from build123d import *

# Parameters (mm, degrees)
SKETCH1_R                = 4.8387
BOSS_EXTRUDE1_DEPTH      = 25.9588
BOSS_EXTRUDE1_DEPTH_BACK = 25.9588
SKETCH2_R                = 4.8387
BOSS_EXTRUDE2_DEPTH      = 6.04901
BOSS_EXTRUDE2_DEPTH_BACK = 6.04901
SKETCH3_R                = 3.2258
CUT_EXTRUDE1_DEPTH       = 13.09802


with BuildPart() as part:
    # Sketch1 → Boss-Extrude1 (new body, two sides)
    with BuildSketch(Plane(origin=(0, 0, 0), x_dir=(0, 0, -1), z_dir=(1, 0, 0))) as boss_extrude1_sk:
        Circle(SKETCH1_R)
    extrude(amount=BOSS_EXTRUDE1_DEPTH)
    extrude(boss_extrude1_sk.sketch, amount=-BOSS_EXTRUDE1_DEPTH_BACK)

    # Sketch2 → Boss-Extrude2 (add, two sides)
    with BuildSketch(Plane.XY) as boss_extrude2_sk:
        with Locations((25.9588, 0)):
            Circle(SKETCH2_R)
        with Locations((-25.9588, 0)):
            Circle(SKETCH2_R)
    extrude(amount=BOSS_EXTRUDE2_DEPTH)
    extrude(boss_extrude2_sk.sketch, amount=-BOSS_EXTRUDE2_DEPTH_BACK)

    # Sketch3 → Cut-Extrude1 (cut, through all)
    with BuildSketch(Plane.XY.offset(6.04901)):
        with Locations((-25.9588, 0)):
            Circle(SKETCH3_R)
        with Locations((25.9588, 0)):
            Circle(SKETCH3_R)
    extrude(amount=-CUT_EXTRUDE1_DEPTH, mode=Mode.SUBTRACT)


solid = part.part
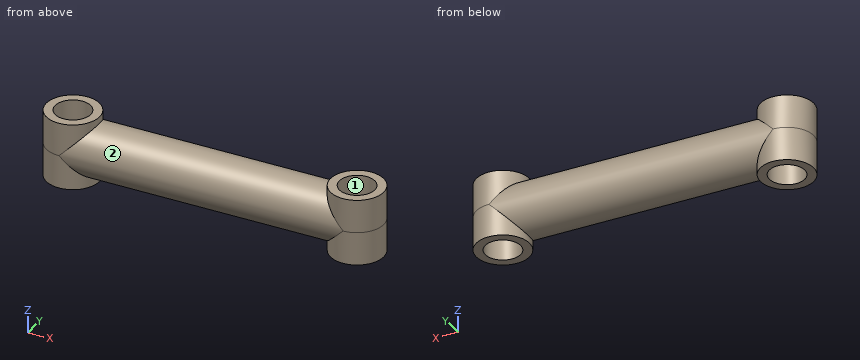
Read the model definition and answer for the solid it produces. Units are mm, in the model's axes. Face numbers are marked on the shaded views. A direction names the side the tool comes from. Coordinates: 2 decimals unless noted, no trailing zeros. Order: outer loops, then holes, each group sorted by start corner. A loop starts at its lowest first (then second) coordinate and runs counter-clockwise, first axis right, second up. Notation, with made-up numbers: (31.25, 89) -> (37.25, 89) arc R4 cw to (37.25, 95) -> close; hole circle Ø1 at (41, 58). An arc over 180 degrees is marked (long way). Answer as a JSON object with one key per item and string values.
1) A cutting plane is placed at C-C, the plane y = 4.25. Determine the outline of the cut face in (x, z).
Model answer:
{"outline": "(-28.27, -6.05) -> (-23.65, -6.05) -> (-23.65, -2.31) -> (23.65, -2.31) -> (23.65, -6.05) -> (28.27, -6.05) -> (28.27, 6.05) -> (23.65, 6.05) -> (23.65, 2.31) -> (-23.65, 2.31) -> (-23.65, 6.05) -> (-28.27, 6.05) -> close"}
2) A cutting plane is placed at D-D, the plane x = -13. Determine the outline of the cut face in (y, z), plus the area to 3 significant figures.
Model answer:
{"outline": "circle Ø9.68 at (0, 0)", "area": "73.6 mm²"}
3) A cutting plane is placed at B-B, the plane z = 2.25. Determine the outline of the cut face in (x, y), plus the area to 3 significant figures.
Model answer:
{"outline": "(-23.71, -4.28) -> (23.71, -4.28) arc R4.84 ccw (long way) to (23.71, 4.28) -> (-23.71, 4.28) arc R4.84 ccw (long way) to start; hole circle Ø6.45 at (-25.96, 0); hole circle Ø6.45 at (25.96, 0)", "area": "456 mm²"}
4) A cutting plane is placed at A-A, the plane y = 0. Determine the outline of the cut face in (x, z).
Model answer:
{"outline": "(-30.8, -6.05) -> (-29.18, -6.05) -> (-29.18, 6.05) -> (-30.8, 6.05) -> close; (-22.73, -6.05) -> (-21.12, -6.05) -> (-21.12, -4.84) -> (21.12, -4.84) -> (21.12, -6.05) -> (22.73, -6.05) -> (22.73, 6.05) -> (21.12, 6.05) -> (21.12, 4.84) -> (-21.12, 4.84) -> (-21.12, 6.05) -> (-22.73, 6.05) -> close; (29.18, -6.05) -> (30.8, -6.05) -> (30.8, 6.05) -> (29.18, 6.05) -> close"}
5) A tool of negligible diameter and unlimited length cuts with its end or side. For the marked faces 1 and 2, from which of +Z, -Z, +X, -X, +Y, -Y can it reach the whole face along a straight path? Write none if from no direction.
Model answer:
{"face 1": "+Z, -Z", "face 2": "none"}
6) Consider line 1 along Y through (x, z) = (26, 4); line 2 along X through (y, z) = (-2.5, -4); line 3 along X through (y, z) = (1.5, 5). Determine where each line is inside the solid, lowest interval first. Write a range as from..to.
Model answer:
{"line 1": "y = -4.84..-3.23, 3.23..4.84", "line 2": "x = -30.1..-28, -23.92..23.92, 28..30.1", "line 3": "x = -30.56..-28.81, -23.1..-21.36, 21.36..23.1, 28.81..30.56"}
7) This flat-tipped pin is pushed along its axis until it touches: pin 1 (3 mm diameter, centred on x = 8, y = 3.5, fed in from -Z). Where does it stop, or does it pass through?
Model answer:
{"pin 1": "stops at z = -4.41"}
